Can you work these out from the model? Positions are in its coordinate system, mm. A direction names the side the tool comes from. Give positions to 0.01 mm unless a question says otherwise; leave off trailing zeros. Loops run counter-clockwise (first coordinate to the right, second up) from the corner with the lowest first, then second, coordinate; pieces in that order, holes last. Notation, with made-up numbers: M 53,-24 L 99,-24 A24 cw 99,-2 Z; hole C 46.25,-35.5 d5. An arc over 180 degrees is marked long. Put each result on its own line as item: value. Start each with the question number.
1) Imagine slicing it at C-C (x = 2). Write out the boundary of the cut face in (y, z), then the cut area to 3 significant figures.
2) Please list where these lines run through material, in increasing order: line 1 along Y through (x, z) = (4.75, 0); line 2 along X through (y, z) = (-4.5, -4); line 3 along X through (y, z) = (-0.5, 6.75). Write a range as from..to.
3) Imagine slicing it at B-B (x = 4.5). Write out the boundary of the cut face in (y, z).
4) If we mould it in two halves opening along X, with no side actions, what happens to faces 5 (the flat face through (11, -5.6, 3)), 6 (the cylindrical face through (12.7, -0.1, -5)), 7 (the flat face through (13.2, 2, -5)), 8 (the flat face through (11, 5.6, 3))? For each: +X half, -X half, draft (parallel to the pull), parting line (faces both ways), or undercut.
5) For P1, Ø2, axis at x = 4.5, z = 2.5, coming from the -Y side; P2, Ø0.8, axis at x = 9.5, z = 2.5, coming from the +Y side (3 decimals); P3, Ø0.5, axis at x = 12.5, y = -6, coming from the +Z side; P4, Ø4, axis at y = 0, z = 0, coming from the -X side, each with a flat end and sliding along its axis, tell me the tip position at first contact or that it passes through.
6) For faces 1 (the flat face through (10.2, -3, -2)), 2 (the flat face through (10, 3.25, 4)), 3 (the cylindrical face through (1.48, 6.21, 3.23)), 4 (the flat face through (12, 6, 6.5)), which set-ups out of +Z, -Z, +X, -X, +Y, -Y let a thin tool reach every point of the face, with its end or its side?
7) Imagine slicing it at A-A (y = 0). Write out the boundary of the cut face in (x, z).
from build123d import *

# Parameters (mm, degrees)
ESBO_O5_W                  = 9.579663193
ESBO_O5_H                  = 10
CORTE_EXTRUS_O3_DEPTH      = 1.5
CORTE_EXTRUS_O4_START      = 2
CORTE_EXTRUS_O4_DEPTH      = 2
ESBO_O8_W                  = 9.704276698
ESBO_O8_H                  = 6.5
CORTE_EXTRUS_O5_DEPTH      = 1
CHANFRO2_SIZE              = 0.2
CHANFRO3_SIZE              = 0.1
CHANFRO4_SIZE              = 0.1
CHANFRO5_SIZE              = 1.5
CORTE_EXTRUS_O6_DEPTH      = 19.834542734
CORTE_EXTRUS_O6_DEPTH_BACK = 19.834542734


with BuildPart() as part:
    # Esboço1 → Revolução1 (revolve)
    with BuildSketch(Plane.XY, mode=Mode.PRIVATE) as revolu_o1_sk:
        Polygon((0, 3.25), (10.2, 3.25), (10.2, 5.6), (12.2, 5.6), (12.2, 5), (13.2, 5), (13.2, 9.5), (6.6, 9.5), (6.6, 5.2), (3.2, 5.2), (3.2, 7), (0, 7), align=None)
    revolve(revolu_o1_sk.sketch.rotate(Axis((0, 0, 0), (1, 0, 0)), 90), axis=Axis((0, 0, 0), (1, 0, 0)))

    # Esboço5 → Corte-extrusão3 (cut)
    with BuildSketch(Plane(origin=(13.2, 0, 0), x_dir=(0, 0, -1), z_dir=(1, 0, 0))):
        with Locations((-4.789831597, 0)):
            Rectangle(ESBO_O5_W, ESBO_O5_H)
    extrude(amount=-CORTE_EXTRUS_O3_DEPTH, mode=Mode.SUBTRACT)

    # Esboço7 → Corte-extrusão4 (cut)
    with BuildSketch(Plane(origin=(10.2, 0, 0), x_dir=(0, 0, -1), z_dir=(1, 0, 0)).offset(CORTE_EXTRUS_O4_START)):
        with BuildLine():
            Line((-9.610816569, -5.6), (0, -5.6))
            ThreePointArc((0, -5.6), (-5.6, 0), (0, 5.6))
            Line((0, 5.6), (-9.610816569, 5.6))
            Line((-9.610816569, 5.6), (-9.610816569, -5.6))
        make_face()
    extrude(amount=-CORTE_EXTRUS_O4_DEPTH, mode=Mode.SUBTRACT)

    # Esboço8 → Corte-extrusão5 (cut)
    with BuildSketch(Plane(origin=(10.2, 0, 0), x_dir=(0, 0, -1), z_dir=(1, 0, 0))):
        with Locations((-4.852138349, 0)):
            Rectangle(ESBO_O8_W, ESBO_O8_H)
    extrude(amount=-CORTE_EXTRUS_O5_DEPTH, mode=Mode.SUBTRACT)

    # Chanfro2
    chanfro2_edges = [part.edges().sort_by_distance(p)[0] for p in [
        (3.2, 0, -7),
    ]]
    chamfer(chanfro2_edges, length=CHANFRO2_SIZE)

    # Chanfro3
    chanfro3_edges = [part.edges().sort_by_distance(p)[0] for p in [
        (13.2, 0, -9.5),
    ]]
    chamfer(chanfro3_edges, length=CHANFRO3_SIZE)

    # Chanfro4
    chanfro4_edges = [part.edges().sort_by_distance(p)[0] for p in [
        (13.2, 5, 3.979949748),
        (13.2, -5, 3.979949748),
        (13.2, 0, -5),
    ]]
    chamfer(chanfro4_edges, length=CHANFRO4_SIZE)

    # Chanfro5
    chanfro5_edges = [part.edges().sort_by_distance(p)[0] for p in [
        (0, 0, -3.25),
    ]]
    chamfer(chanfro5_edges, length=CHANFRO5_SIZE)

    # Esboço9 → Corte-extrusão6 (cut, two sides: drawn at the far end of the back side and taken through both)
    with BuildSketch(Plane(origin=(0, 0, 0), x_dir=(1, 0, 0), z_dir=(0, 1, 0)).offset(-CORTE_EXTRUS_O6_DEPTH_BACK)):
        with BuildLine():
            Line((11.6, -6.5), (13.2, -6.5))
            Line((13.2, -6.5), (13.2, -12.5))
            Line((13.2, -12.5), (11.6, -12.5))
            ThreePointArc((11.6, -12.5), (8.6, -9.5), (11.6, -6.5))
        make_face()
    extrude(amount=CORTE_EXTRUS_O6_DEPTH + CORTE_EXTRUS_O6_DEPTH_BACK, mode=Mode.SUBTRACT)


solid = part.part
Recorded:
1. outline: C 0,0 d14; hole C 0,0 d6.5
1. area: 121 mm²
2. line 1: -5.2..-3.25, 3.25..5.2
2. line 2: 0..3.2, 6.6..13.2
2. line 3: 0..3.2, 6.6..9.2
3. outline: C 0,0 d10.4; hole C 0,0 d6.5
4. face 5: undercut
4. face 6: draft
4. face 7: +X half
4. face 8: undercut
5. P1: y = -4.98
5. P2: y = 9.265
5. P3: z = 6.5
5. P4: through
6. face 1: +Z
6. face 2: +Z, +X
6. face 3: -X
6. face 4: +Z, +X, +Y, -Y
7. outline: M 0,-7 L 3,-7 L 3.2,-6.8 L 3.2,-5.2 L 6.6,-5.2 L 6.6,-9.5 L 13.1,-9.5 L 13.2,-9.4 L 13.2,-5.1 L 13.1,-5 L 12.2,-5 L 12.2,-5.6 L 10.2,-5.6 L 10.2,-3.25 L 1.5,-3.25 L 0,-4.75 Z; M 0,4.75 L 1.5,3.25 L 9.2,3.25 L 9.2,7.7 A3 cw 8.6,9.5 L 6.6,9.5 L 6.6,5.2 L 3.2,5.2 L 3.2,6.8 L 3,7 L 0,7 Z
